Autodesk Inventor part; units mm, degrees
ref_plane "YZ Plane" through (0, 0, 0) normal (1, 0, 0) x (0, 1, 0)
ref_plane "XZ Plane" through (0, 0, 0) normal (0, 1, 0) x (-1, 0, 0)
ref_plane "XY Plane" through (0, 0, 0) normal (0, 0, 1) x (1, 0, 0)
sketch "Sketch1" plane through (0, 0, 0) normal (0, 0, 1) x (1, 0, 0)
  line L0 (-4.9459, 24.2237) -> (10.0541, 24.2237)
  line L1 (10.0541, 24.2237) -> (10.0541, -0.7763)
  line L2 (10.0541, -0.7763) -> (-4.9459, -0.7763)
  line L3 (-4.9459, -0.7763) -> (-4.9459, 24.2237)
  point P0 (0, 0)
  dimension "d0" = 15
  dimension "d1" = 25
extrude "Extrusion1" add sketch "Sketch1" along normal blind 15
fillet "Fillet1" radius 2 12 edges at (10.0541, 11.7237, 15) (10.0541, 24.2237, 7.5) (10.0541, 11.7237, 0) (10.0541, -0.7763, 7.5) (2.5541, -0.7763, 15) (2.5541, 24.2237, 15) (2.5541, 24.2237, 0) (2.5541, -0.7763, 0) (-4.9459, 24.2237, 7.5) (-4.9459, 11.7237, 15) (-4.9459, -0.7763, 7.5) (-4.9459, 11.7237, 0)
sketch "Sketch2" plane through (-4.9459, 1.2237, 13) normal (-1, 0, 0) x (0, 0, 1)
  line L0 (-9.7554, 1.003) -> (-9.7554, 19.8346)
  line L1 (-11, 0) -> (-11, 21)
  line L2 (-9.7554, 19.8346) -> (-0.9757, 19.8346)
  line L3 (-0.9757, 19.8346) -> (-0.9757, 1.003)
  line L4 (-0.9757, 1.003) -> (-9.7554, 1.003)
  point P0 (-13, -1.2237)
extrude "Extrusion2" cut sketch "Sketch2" against normal blind 14
sketch "Sketch3" plane through (0, 0, 15) normal (0, 0, 1) x (1, 0, 0)
  line L0 (8.0541, 22.2237) -> (8.0541, 1.2237)
  line L1 (0, 8.0798) -> (8.0541, 8.0798)
  line L2 (8.0541, 8.0798) -> (8.0541, 15.7143)
  line L3 (8.0541, 15.7143) -> (0, 15.7143)
  line L4 (0, 15.7143) -> (0, 8.0798)
  point P0 (0, 0)
extrude "Extrusion3" cut sketch "Sketch3" against normal blind 14
sketch "Sketch4" plane through (-4.9459, 1.2237, 13) normal (-1, 0, 0) x (0, 0, 1)
  circle A0 centre (-5.5, 22.1852) radius 0.75
  point P0 (-13, -1.2237)
  dimension "d9" = 1.5
extrude "Extrusion4" add sketch "Sketch4" against normal blind 15
sketch "Sketch5" plane through (9.0541, 1.2237, 13) normal (-1, 0, 0) x (0, 0, 1)
  circle A0 centre (-8.6725, -1.2237) radius 0.75
  point P0 (-13, -1.2237)
  dimension "d12" = 1.5
extrude "Extrusion5" cut sketch "Sketch5" against normal blind 15
sketch "Sketch6" plane through (9.0541, 1.2237, 13) normal (-1, 0, 0) x (0, 0, 1)
  circle A0 centre (-5.5, -1.2237) radius 0.75
  point P0 (-13, -1.2237)
  dimension "d15" = 1.5
extrude "Extrusion6" add sketch "Sketch6" along normal blind 2
sketch "Sketch7" plane through (-4.9459, 2.2267, 12.0243) normal (0, 1, 0) x (1, 0, 0)
  point P0 (4.9459, 12.0243)
sketch "Sketch8" plane through (-4.9459, 1.2237, 13) normal (-1, 0, 0) x (0, 0, 1)
  circle A0 centre (-5.7946, -1.2237) radius 0.75
  point P0 (-13, -1.2237)
  dimension "d18" = 1.5
extrude "Extrusion7" add sketch "Sketch8" against normal blind 14
properties part number "F5"
Design review of the part built by this model. Coordinates are the model's own, in mm. A direction names the side the tool comes from. Coordinates: 2 decimals unless noted, no trailing zeros. Order: outer loops, then holes, each group sorted by start corner. A loop starts at its lowest first (then second) coordinate and runs counter-clockwise, first axis right, second up. Notation, with made-up numbers: (2.25, 20) -> (15.25, 20) arc R23 cw to (15.25, 50) -> close; hole circle Ø3 at (65.25, -12.75). An arc over 180 degrees is marked (long way). One line per item, written item: value.
1) Clearance check with flat-ended pins moving along their axes: P1, Ø0.9, axis at y = 0, z = 4.33, coming from the +X side; P2, Ø0.7, axis at y = 13, z = 1.5, coming from the -X side; P3, Ø4.5, axis at y = 13, z = 8, coming from the -X side. State where each tip first meets the part, or that it passes through.
Output values:
P1: stops at x = 9.05
P2: stops at x = -4.94
P3: stops at x = 9.05
2) Machinability: for faces 1 (the face through (4, 12, 1)), 2 (the face through (-4.376, 11.871, 14.399)), 3 (the face through (-1, 12, 3.245)), which of the approach directions +Z, -Z, +X, -X, +Y, -Y give a long, thin tool a straight path to every point of the face, cutting with its end or side? Answer none if there is none.
Output values:
face 1: +Z
face 2: +Z, -X, +Y, -Y
face 3: -X
3) To check wall thickness, follow probe 1 along Z at (x, y) = (8, 17); probe 2 along Y at (x, z) = (7.5, 9.5); probe 3 along Y at (x, z) = (3.5, 12.5). State the ranges of each line that lie inside material, in increasing order. Write a range as [from, to].
Output values:
probe 1: z = [0, 3.24], [12.02, 15]
probe 2: y = [-0.78, 2.23], [21.06, 24.22]
probe 3: y = [-0.78, 8.08], [15.71, 24.22]
4) We need section B-B, the plane x = 1. Give the boundary of the cut face in (y, z), then the cut area to 3 significant figures.
Output values:
outline: (-0.78, 2) arc R2 ccw to (1.22, 0) -> (22.22, 0) arc R2 ccw to (24.22, 2) -> (24.22, 13) arc R2 ccw to (22.22, 15) -> (15.71, 15) -> (15.71, 12.02) -> (21.06, 12.02) -> (21.06, 3.24) -> (15.71, 3.24) -> (15.71, 1) -> (8.08, 1) -> (8.08, 3.24) -> (2.23, 3.24) -> (2.23, 12.02) -> (8.08, 12.02) -> (8.08, 15) -> (1.22, 15) arc R2 ccw to (-0.78, 13) -> close
area: 166 mm2
5) We need section A-A, the plane y = 14. Give the boundary of the cut face in (x, z), then the cut area to 3 significant figures.
Output values:
outline: (-4.95, 2) arc R2 ccw to (-2.95, 0) -> (8.05, 0) arc R2 ccw to (10.05, 2) -> (10.05, 13) arc R2 ccw to (8.05, 15) -> (8.05, 12.02) -> (9.05, 12.02) -> (9.05, 3.24) -> (8.05, 3.24) -> (8.05, 1) -> (0, 1) -> (0, 3.24) -> (-4.95, 3.24) -> close; (-4.95, 12.02) -> (0, 12.02) -> (0, 15) -> (-2.95, 15) arc R2 ccw to (-4.95, 13) -> close
area: 56.6 mm2
6) We need section D-D, the plane z = 2.5. Give the boundary of the cut face in (x, y).
Output values:
outline: (-4.95, 1.22) arc R2 ccw to (-2.95, -0.78) -> (8.05, -0.78) arc R2 ccw to (10.05, 1.22) -> (10.05, 22.22) arc R2 ccw to (8.05, 24.22) -> (-2.95, 24.22) arc R2 ccw to (-4.95, 22.22) -> close; hole (0, 8.08) -> (8.05, 8.08) -> (8.05, 15.71) -> (0, 15.71) -> close
7) Draft analysis for pull direction X (two halves, no side actions). For faces 4 (the face through (0, 12, 2)), 5 (the face through (2, 21.058, 8)), 6 (the face through (8.054, 12, 2)), 7 (the face through (9.484, 23.622, 6.355)), state which applies: +X half, -X half, draft (parallel to the pull), parting line (faces both ways), or undercut.
Output values:
face 4: undercut
face 5: draft
face 6: undercut
face 7: +X half
8) We need section C-C, the plane z = 11.25. Give the boundary of the cut face in (x, y).
Output values:
outline: (-4.95, 1.22) arc R2 ccw to (-2.95, -0.78) -> (8.05, -0.78) arc R2 ccw to (10.05, 1.22) -> (10.05, 22.22) arc R2 ccw to (8.05, 24.22) -> (-2.95, 24.22) arc R2 ccw to (-4.95, 22.22) -> (-4.95, 21.06) -> (9.05, 21.06) -> (9.05, 2.23) -> (-4.95, 2.23) -> close
